For this review, take the finished solid that the model builds, in its own axes (mm). Round coordinates to 2 decimals unless told otherwise and drop trailing zeros. Write each loop counter-clockwise with the first axis right and the second up, starting at its lowest first coordinate (ties: lowest second). Pieces come first, ordered by that corner, then holes. Notation, with made-up numbers: (81.25, 42) - (130.25, 42) arc R18 cw to (130.25, 55) - close; hole circle Ø10 at (58.25, 41). An arc over 180 degrees is marked (long way). Answer in a Markdown table with one row per item. Add a question column.
from build123d import *

# Parameters (mm, degrees)
SKETCH1_R             = 49.4665
BOSS_EXTRUDE1_DEPTH   = 6.35
F_3_0MM_DOWEL_HOLE1_D = 3
SKETCH5_R             = 3.175
CUT_EXTRUDE1_DEPTH    = 71.243802179
SKETCH6_R             = 3.175
CUT_EXTRUDE2_DEPTH    = 71.243802179
SKETCH7_R             = 11.049
CUT_EXTRUDE3_DEPTH    = 71.243802179


with BuildPart() as part:
    # Sketch1 → Boss-Extrude1 (new body)
    with BuildSketch(Plane.XY):
        Circle(SKETCH1_R)
    extrude(amount=BOSS_EXTRUDE1_DEPTH)

    # Ø3.0mm Dowel Hole1 (through all)
    with Locations(Plane.XY.offset(6.35)):
        with Locations((15.5, 0.26), (-15.5, 0.26), (-15.5, -30.74), (15.5, -30.74)):
            Hole(F_3_0MM_DOWEL_HOLE1_D / 2)

    # Sketch5 → Cut-Extrude1 (cut, through all)
    with BuildSketch(Plane.XY.offset(6.35)):
        with Locations((0, -42.672)):
            Circle(SKETCH5_R)
        with Locations((0, 12.26)):
            Circle(SKETCH5_R)
    extrude(amount=-CUT_EXTRUDE1_DEPTH, mode=Mode.SUBTRACT)

    # Sketch6 → Cut-Extrude2 (cut, through all)
    with BuildSketch(Plane.XY.offset(6.35)):
        with Locations((0, 38.128211777)):
            Circle(SKETCH6_R)
        with Locations((-33.02, -19.064105889)):
            Circle(SKETCH6_R)
        with Locations((33.02, -19.064105889)):
            Circle(SKETCH6_R)
    extrude(amount=-CUT_EXTRUDE2_DEPTH, mode=Mode.SUBTRACT)

    # Sketch7 → Cut-Extrude3 (cut, through all)
    with BuildSketch(Plane.XY.offset(6.35)):
        with Locations((0, -15.24)):
            Circle(SKETCH7_R)
    extrude(amount=-CUT_EXTRUDE3_DEPTH, mode=Mode.SUBTRACT)


solid = part.part
Q1. Insertion check: pin 1 Ø1 at (y, z) = (-23, 3) entering from -X. The pin has a flat end and moves straight along its axis. Give the tip position at first contact, or say it passes through.
Q2. To check wall thickness, follow probe 1 along Y at (x, z) = (0, 4) (1 decimal); probe 2 along Y at (x, z) = (1.5, 3); probe 3 along Y at (x, z) = (-15.5, 3.25). State the ranges of each line that lie inside material, in increasing order.
Q3. Draft analysis for pull direction Y (two halves, no side actions). For faces 1 (the face through (-1, 1, 6.35)), 2 (the face through (47.18, 14.86, 3.13)), 3 (the face through (-0.413, 41.276, 3.219)), 4 (the face through (-0.69, -45.77, 3.22)), state which applies: released by +Y, released by -Y, zero draft, split by the parting line, or undercut.
Q4. Add section D-D on y = 29.5. State the section outline as (x, z) points, then the cut area to 3 significant figures.
Q5. Add section C-C on z = 2. Count the separate pieces of the cut face and the enclosed holes in it, then the cut area to 3 significant figures.
Q6. Add section B-B on y = -11.5. State the section outline as (x, z) points, then the cut area to 3 significant figures.
Q7. Add section A-A on x = 8. State the section outline as (y, z) points.
Answer sheet:
| question | item | result |
|---|---|---|
| 1 | pin 1 | stops at x = -44.05 |
| 2 | probe 1 | y = -49.5 to -45.8, -39.5 to -26.3, -4.2 to 9.1, 15.4 to 35, 41.3 to 49.5 |
| 2 | probe 2 | y = -49.44 to -45.47, -39.87 to -26.19, -4.29 to 9.46, 15.06 to 35.33, 40.93 to 49.44 |
| 2 | probe 3 | y = -46.98 to -32.24, -29.24 to -1.24, 1.76 to 46.98 |
| 3 | face 1 | zero draft |
| 3 | face 2 | split by the parting line |
| 3 | face 3 | undercut |
| 3 | face 4 | undercut |
| 4 | outline | (-39.71, 0) - (39.71, 0) - (39.71, 6.35) - (-39.71, 6.35) - close |
| 4 | area | 504 mm² |
| 5 | separate pieces | 1 |
| 5 | enclosed holes | 10 |
| 5 | area | 7,120 mm² |
| 6 | outline | (-48.11, 0) - (-10.4, 0) - (-10.4, 6.35) - (-48.11, 6.35) - close; (10.4, 0) - (48.11, 0) - (48.11, 6.35) - (10.4, 6.35) - close |
| 6 | area | 479 mm² |
| 7 | outline | (-48.82, 0) - (-22.86, 0) - (-22.86, 6.35) - (-48.82, 6.35) - close; (-7.62, 0) - (48.82, 0) - (48.82, 6.35) - (-7.62, 6.35) - close |
